```python
from build123d import *

# Parameters (mm, degrees)
SKETCH_1_W          = 15
SKETCH_1_H          = 10
SKETCH_1_W_2        = 12
SKETCH_1_H_2        = 8
EXTRUDE_1_DEPTH     = 40
SKETCH_2_R          = 1.6
CUT_EXTRUDE_1_DEPTH = 44.011626335
SKETCH_4_R          = 1.6
CUT_EXTRUDE_3_DEPTH = 44.011626335
SKETCH_5_R          = 1.6
CUT_EXTRUDE_4_DEPTH = 42.907636536
SKETCH_6_W          = 15
SKETCH_6_H          = 10
SKETCH_6_W_2        = 12
SKETCH_6_H_2        = 8
EXTRUDE_2_DEPTH     = 600
SKETCH_7_R          = 1.6
CUT_EXTRUDE_5_DEPTH = 641.122058673
SKETCH_8_R          = 1.6
CUT_EXTRUDE_6_DEPTH = 641.195282707


with BuildPart() as part:
    # ｽｹｯﾁ1 → ﾎﾞｽ - 押し出し1 (new body)
    with BuildSketch(Plane.XY):
        Rectangle(SKETCH_1_W, SKETCH_1_H)
        Rectangle(SKETCH_1_W_2, SKETCH_1_H_2, mode=Mode.SUBTRACT)
    extrude_1 = extrude(amount=EXTRUDE_1_DEPTH)

    # ｽｹｯﾁ2 → ｶｯﾄ - 押し出し1 (cut, through all)
    with BuildSketch(Plane(origin=(7.5, 0, 0), x_dir=(0, 0, -1), z_dir=(1, 0, 0))):
        with Locations((-20, 0)):
            Circle(SKETCH_2_R)
    cut_extrude_1 = extrude(amount=-CUT_EXTRUDE_1_DEPTH, mode=Mode.SUBTRACT)

    # ｽｹｯﾁ4 → ｶｯﾄ - 押し出し3 (cut, through all)
    with BuildSketch(Plane.ZY.offset(7.5)):
        with Locations((35, 0)):
            Circle(SKETCH_4_R)
    cut_extrude_3 = extrude(amount=-CUT_EXTRUDE_3_DEPTH, mode=Mode.SUBTRACT)

    # ｽｹｯﾁ5 → ｶｯﾄ - 押し出し4 (cut, through all)
    with BuildSketch(Plane(origin=(0, 5, 0), x_dir=(1, 0, 0), z_dir=(0, 1, 0))):
        with Locations(Location((0, -25, 0), (0, 0, 270))):
            Circle(SKETCH_5_R)
    cut_extrude_4 = extrude(amount=-CUT_EXTRUDE_4_DEPTH, mode=Mode.SUBTRACT)

    # ﾐﾗｰ1: ﾎﾞｽ - 押し出し1, ｶｯﾄ - 押し出し1, ｶｯﾄ - 押し出し3, ｶｯﾄ - 押し出し4 across plane
    add(extrude_1.mirror(Plane(origin=(0, 0, 0), x_dir=(1, 0, 0), z_dir=(0, 0, -1))))
    add(cut_extrude_1.mirror(Plane(origin=(0, 0, 0), x_dir=(1, 0, 0), z_dir=(0, 0, -1))), mode=Mode.SUBTRACT)
    add(cut_extrude_3.mirror(Plane(origin=(0, 0, 0), x_dir=(1, 0, 0), z_dir=(0, 0, -1))), mode=Mode.SUBTRACT)
    add(cut_extrude_4.mirror(Plane(origin=(0, 0, 0), x_dir=(1, 0, 0), z_dir=(0, 0, -1))), mode=Mode.SUBTRACT)

    # ｽｹｯﾁ6 → ﾎﾞｽ - 押し出し2 (add)
    with BuildSketch(Plane(origin=(0, 0, -40), x_dir=(-1, 0, 0), z_dir=(0, 0, -1))):
        Rectangle(SKETCH_6_W, SKETCH_6_H)
        Rectangle(SKETCH_6_W_2, SKETCH_6_H_2, mode=Mode.SUBTRACT)
    extrude(amount=EXTRUDE_2_DEPTH)

    # ｽｹｯﾁ7 → ｶｯﾄ - 押し出し5 (cut, through all)
    with BuildSketch(Plane(origin=(0, -5, 0), x_dir=(-1, 0, 0), z_dir=(0, -1, 0))):
        with Locations(Location((0, 635, 0), (0, 0, 90))):
            Circle(SKETCH_7_R)
        with Locations(Location((0, 80, 0), (0, 0, 90))):
            Circle(SKETCH_7_R)
        with Locations(Location((0, 70, 0), (0, 0, 90))):
            Circle(SKETCH_7_R)
        with Locations(Location((0, 475, 0), (0, 0, 90))):
            Circle(SKETCH_7_R)
    extrude(amount=-CUT_EXTRUDE_5_DEPTH, mode=Mode.SUBTRACT)

    # ｽｹｯﾁ8 → ｶｯﾄ - 押し出し6 (cut, through all)
    with BuildSketch(Plane(origin=(7.5, 0, 0), x_dir=(0, 0, -1), z_dir=(1, 0, 0))):
        with Locations((330, 0)):
            Circle(SKETCH_8_R)
        with Locations((580, 0)):
            Circle(SKETCH_8_R)
        with Locations((180, 0)):
            Circle(SKETCH_8_R)
        with Locations((250, 0)):
            Circle(SKETCH_8_R)
        with Locations((560, 0)):
            Circle(SKETCH_8_R)
        with Locations((620, 0)):
            Circle(SKETCH_8_R)
    extrude(amount=-CUT_EXTRUDE_6_DEPTH, mode=Mode.SUBTRACT)


solid = part.part
```
Here's how the part is built. I have some questions about the finished solid (model axes, mm). A direction names the side the tool comes from. Coordinates: 2 decimals unless noted, no trailing zeros. Loops run counter-clockwise (first coordinate to the right, second up) from the corner with the lowest first, then second, coordinate; pieces in that order, holes last. Notation, with made-up numbers: M -22.5,86 L 16.5,86 A29 ccw 16.5,118 Z; hole C -30.5,-28.75 d1. An arc over 180 degrees is marked long. One line per item, written item: value.
1. Thinking about a two-plate mould opening in X: for faces 3 (the flat face through (0, -4, -295)), 4 (the flat face through (0, -5, -295)), which applies, +X half, -X half, draft (parallel to the pull), parting line (faces both ways), or undercut?
Geometry says:
face 3: undercut
face 4: draft
2. Imagine slicing it at A-A (z = -383). List the corners of the cut face in (x, y) for me.
Geometry says:
outline: M -7.5,-5 L 7.5,-5 L 7.5,5 L -7.5,5 Z; hole M -6,-4 L 6,-4 L 6,4 L -6,4 Z
3. Please list where these lines run through material, in increasing order: probe 1 along Y at (x, z) = (-0.75, -254); probe 2 along X at (y, z) = (3.5, -86); probe 3 along X at (y, z) = (-4.25, -635).
Geometry says:
probe 1: y = -5 to -4, 4 to 5
probe 2: x = -7.5 to -6, 6 to 7.5
probe 3: x = -7.5 to -1.6, 1.6 to 7.5
4. Will these pins go through, and if not, where does the flat tip stop? pin 1 Ø5 at (x, z) = (0, 25) entering from +Y; pin 2 Ø1.9 at (x, z) = (0, -635) entering from -Y.
Geometry says:
pin 1: stops at y = 5
pin 2: passes through
5. Imagine slicing it at B-B (y = 0). State how many separate pieces and enclosed holes the cut face has, and give its area (3 significant figures).
Geometry says:
separate pieces: 22
enclosed holes: 0
area: 1,940 mm2
6. On a 3-axis mill with a long thin cutter (end or side, diameter ignored), from which of +Z, -Z, +X, -X, +Y, -Y can I reach the whole of each face in a straight line? I mean faces 1 (the flat face through (0, 4, -295)), 2 (the flat face through (0, 5, -295)). Say none if no direction works.
Geometry says:
face 1: +Z, -Z
face 2: +Z, -Z, +X, -X, +Y
